```python
from build123d import *

# Parameters (mm, degrees)
F1_R          = 3
F2_DEPTH      = 15
F1_R_2        = 5
F3_DEPTH      = 10
F3_DEPTH_BACK = 8.58
F4_S5_R       = 3
F4_T6_DEPTH   = 13095
F6_DEPTH      = 9.05
F7_R          = 3
F8_DEPTH      = 25
F8_DEPTH_BACK = 25


# Not quite as in the source:
# - a fillet or chamfer that OpenCascade refuses, or shapes differently, is made with other operations: its cross-section is extruded or revolved along the edge and cut away or added


with BuildPart() as f2:
    # F1 (on Front) → F2 (new body)
    with BuildSketch(Plane.XZ):
        Circle(F1_R)
    extrude(amount=F2_DEPTH)

    # F1 (on Front) → F3 (join, two sides)
    with BuildSketch(Plane.XZ) as f3_sk:
        Circle(F1_R_2)
        Circle(F1_R, mode=Mode.SUBTRACT)
        Circle(F1_R)
    extrude(amount=-F3_DEPTH)
    extrude(f3_sk.sketch, amount=F3_DEPTH_BACK)

    # F4: fillet of radius 5 on 1 edges, made by hand


with BuildPart() as f4_tool2:
    # F4_s3 → F4_t4 (revolve)
    with BuildSketch(Plane.XY):
        with BuildLine():
            ThreePointArc((0, -8.5803999068), (3.5358753108, -7.1151924681), (5.0004, -3.5790343146))
            Line((5.0004, -3.5790343146), (5.5005365685, -3.5790343146))
            ThreePointArc((5.5005365685, -3.5790343146), (5.5001365685, -6.0795171573), (5.5001365685, -8.58))
            Line((5.5001365685, -8.58), (5, -9.0801365685))
            Line((5, -9.0801365685), (0, -9.0805364913))
            Line((0, -9.0805364913), (0, -8.5803999068))
        make_face()
    revolve(axis=Axis((0, -8.58, 0), (0, -1, 0)))

    # F4_s5 → F4_t6 (cut, symmetric)
    with BuildSketch(Plane.XZ.offset(7.3)):
        Circle(F4_S5_R)
    extrude(amount=F4_T6_DEPTH, both=True, mode=Mode.SUBTRACT)


with BuildPart() as f2_1:
    add(f2.part)

    # F4_t1: cut F4_tool2
    add(f4_tool2.part, mode=Mode.SUBTRACT)

    # F5 (on face) → F6 (cut)
    with BuildSketch(Plane(origin=(0, 10, 0), x_dir=(-1, 0, 0), z_dir=(0, 1, 0))):
        with BuildLine():
            Line((-2, 4.582575695), (-2, -4.582575695))
            ThreePointArc((-2, -4.582575695), (0, -5), (2, -4.582575695))
            Line((2, -4.582575695), (2, 4.582575695))
            ThreePointArc((2, 4.582575695), (0, 5), (-2, 4.582575695))
        make_face()
    extrude(amount=-F6_DEPTH, mode=Mode.SUBTRACT)

    # F7 (on face) → F8 (cut, two sides)
    with BuildSketch(Plane.YZ.offset(-2)) as f8_sk:
        with Locations((6, 0)):
            Circle(F7_R)
    extrude(amount=F8_DEPTH, mode=Mode.SUBTRACT)
    extrude(f8_sk.sketch, amount=-F8_DEPTH_BACK, mode=Mode.SUBTRACT)

    # F9: F2 across face


with BuildPart() as f2_2:
    add(f2_1.part)
    add(f2_1.part.mirror(Plane.XZ.offset(15)))


solid = f2_2.part
```
Here's how the part is built. I have some questions about the finished solid (model axes, mm). A direction names the side the tool comes from. Coordinates: 2 decimals unless noted, no trailing zeros. Order: outer loops, then holes, each group sorted by start corner. A loop starts at its lowest first (then second) coordinate and runs counter-clockwise, first axis right, second up.
1) We'd pull the mould along X, two halves only. Please class faces 1 (the face through (2, -33.5, 2.1)), 2 (the face through (4.619, 1.759, -1.915)), 3 (the face through (3, 10, 0)): +X half, -X half, draft (parallel to the pull), parting line (faces both ways), or undercut.
2) Will these pins go through, and if not, where does the flat tip stop? pin 1 (1.5 mm diameter, centred on y = 4.5, z = -2.5, fed in from +X); pin 2 (6 mm diameter, centred on y = -10.5, z = -4, fed in from -X); pin 3 (2.5 mm diameter, centred on y = 4, z = 2, fed in from +X).
3) I need wall thicknesses on line 1 (Y direction, x = 2.7, z = 0); line 2 (Y direction, x = -3.2, z = 0); line 3 (X direction, y = -33, z = 4). Which ranges of each line are inside material? Lowest first, please.
4) Imagine slicing it at A-A on y = 6. List the corners of the cut face in (x, z) for me, and give its area (3 significant figures).
5) Which directions (+Z, -Z, +X, -X, +Y, -Y) give clear straight access to the entire face, cutting with the end or side of a thin tool? Please do faces 4 (the face through (0, -30.95, 0)), 5 (the face through (-2, 3.5, -2.1)), 6 (the face through (-3.15, -38.86, 0.9)).
6) Imagine slicing it at B-B on x = 3.5. State how many separate pieces and enclosed holes the cut face has, and give its area (3 significant figures).
7) Imagine slicing it at D-D on y = -28. List the corners of the cut face in (x, z) for me, and give its area (3 significant figures).
Response values:
1. face 1: undercut
1. face 2: parting line
1. face 3: draft
2. pin 1: stops at x = 4.54
2. pin 2: stops at x = -2.83
2. pin 3: stops at x = 4.89
3. line 1: y = -40 to -39, -33 to 3, 9 to 10
3. line 2: y = -40 to -39, -33 to -22.58, -7.42 to 3, 9 to 10
3. line 3: x = -3 to -2, 2 to 3
4. outline: (-4, -3) arc R5 ccw to (-2, -4.58) - (-2, -3) - close; (-4, 3) - (-2, 3) - (-2, 4.58) arc R5 ccw to start; (2, -4.58) arc R5 ccw to (4, -3) - (2, -3) - close; (2, 3) - (4, 3) arc R5 ccw to (2, 4.58) - close
4. area: 7.46 mm2
5. face 4: +Z, -Z, -Y
5. face 5: +Z, -Z, +Y
5. face 6: +X, -X
6. separate pieces: 2
6. enclosed holes: 2
6. area: 177 mm2
7. outline: circle Ø10 at (0, 0)
7. area: 78.5 mm2
